from build123d import *

# Parameters (mm, degrees)
SALIENTE_EXTRUIR3_DEPTH    = 3
SALIENTE_EXTRUIR4_DEPTH    = 37
CROQUIS15_R                = 1.05
CROQUIS15_W                = 14
CROQUIS15_H                = 5.5
CORTAR_EXTRUIR6_DEPTH      = 9
CROQUIS17_W                = 2.75
CROQUIS17_H                = 14
CROQUIS17_R                = 1.05
CORTAR_EXTRUIR7_DEPTH      = 205.947432284
CORTAR_EXTRUIR8_DEPTH      = 200.161793525
CORTAR_EXTRUIR8_DEPTH_BACK = 200.161793525
CROQUIS18_R                = 4.05
CROQUIS18_R_2              = 1.55
CROQUIS20_R                = 1.55
CROQUIS20_R_2              = 4.05
CORTAR_EXTRUIR9_DEPTH      = 5.5
CROQUIS21_W                = 38.703075187
CROQUIS21_H                = 31.902541418
CROQUIS21_R                = 1.55
CROQUIS21_R_2              = 4.05
CORTAR_EXTRUIR11_DEPTH     = 5.5
CROQUIS24_R                = 1.55
CORTAR_EXTRUIR12_DEPTH     = 5.5
SALIENTE_EXTRUIR5_START    = 5.5
CROQUIS25_R                = 3.5
CROQUIS25_R_2              = 1.55
SALIENTE_EXTRUIR5_DEPTH    = 5.5
CROQUIS27_W                = 4.4
CROQUIS27_H                = 9.7
CORTAR_EXTRUIR13_DEPTH     = 191.373895269
CROQUIS28_R                = 1.55
CORTAR_EXTRUIR14_DEPTH     = 5.5


with BuildPart() as part:
    # PacmanSilueta → Saliente-Extruir3 (new body)
    with BuildSketch(Plane.XY):
        Polygon((-79.1, 2.1), (-79.1, -93), (-79.1, -100.1), (-68.1, -100.1), (-68.1, -111.1), (-31.486400432, -111.1), (-31.486400432, -100.1), (-13.1, -100.1), (-13.1, -111.1), (23.1, -111.1), (23.1, -100.1), (41.486400432, -100.1), (41.486400432, -111.1), (78.1, -111.1), (78.1, -100.1), (89.1, -100.1), (89.1, 2.1), (78.1, 2.1), (78.1, 35.1), (67.1, 35.1), (67.1, 46.1), (56.1, 46.1), (56.1, 57.1), (34.1, 57.1), (34.1, 68.1), (-24.1, 68.1), (-24.1, 57.1), (-46.1, 57.1), (-46.1, 46.1), (-57.1, 46.1), (-57.1, 35.1), (-68.1, 35.1), (-68.1, 2.1), align=None)
    extrude(amount=-SALIENTE_EXTRUIR3_DEPTH)

    # Croquis3 → Saliente-Extruir4 (add)
    with BuildSketch(Plane.XY):
        Polygon((-46.1, 46.1), (-57.1, 46.1), (-57.1, 35.1), (-68.1, 35.1), (-68.1, 2.1), (-79.1, 2.1), (-79.1, -100.1), (-68.1, -100.1), (-68.1, -111.1), (-31.486400432, -111.1), (-31.486400432, -100.1), (-13.1, -100.1), (-13.1, -111.1), (23.1, -111.1), (23.1, -100.1), (41.486400432, -100.1), (41.486400432, -111.1), (78.1, -111.1), (78.1, -100.1), (89.1, -100.1), (89.1, 2.1), (78.1, 2.1), (78.1, 35.1), (67.1, 35.1), (67.1, 46.1), (56.1, 46.1), (56.1, 57.1), (34.1, 57.1), (34.1, 68.1), (-24.1, 68.1), (-24.1, 57.1), (-46.1, 57.1), align=None)
        Polygon((-72, -93), (-72, -5), (-61, -5), (-61, 28), (-50, 28), (-50, 39), (-39, 39), (-39, 50), (-17, 50), (-17, 61), (27, 61), (27, 50), (49, 50), (49, 39), (60, 39), (60, 28), (71, 28), (71, -5), (82, -5), (82, -93), (71, -93), (71, -104), (48.586400432, -104), (48.586400432, -93), (16, -93), (16, -104), (-6, -104), (-6, -93), (-38.586400432, -93), (-38.586400432, -104), (-61, -104), (-61, -93), align=None, mode=Mode.SUBTRACT)
    extrude(amount=SALIENTE_EXTRUIR4_DEPTH)

    # Croquis15 → Cortar-Extruir6 (cut)
    with BuildSketch(Plane(origin=(0, 68.1, 0), x_dir=(1, 0, 0), z_dir=(0, 1, 0))):
        with Locations(Location((-15.4, -8.6, 0), (0, 0, 180))):
            Circle(CROQUIS15_R)
        with Locations((-15.4, -25.4)):
            Circle(CROQUIS15_R)
        with Locations(Location((25.4, -8.6, 0), (0, 0, 180))):
            Circle(CROQUIS15_R)
        with Locations(Location((25.4, -25.4, 0), (0, 0, 180))):
            Circle(CROQUIS15_R)
        with Locations((5, -7)):
            Rectangle(CROQUIS15_W, CROQUIS15_H)
    extrude(amount=-CORTAR_EXTRUIR6_DEPTH, mode=Mode.SUBTRACT)

    # Croquis17 → Cortar-Extruir7 (cut, through all)
    with BuildSketch(Plane.ZY.offset(79.1)):
        with Locations((8.375, -29)):
            Rectangle(CROQUIS17_W, CROQUIS17_H)
        with Locations((5.625, -29)):
            Rectangle(CROQUIS17_W, CROQUIS17_H)
        with Locations((25.4, -8.6)):
            Circle(CROQUIS17_R)
        with Locations(Location((8.6, -8.6, 0), (0, 0, 180))):
            Circle(CROQUIS17_R)
        with Locations(Location((25.4, -49.4, 0), (0, 0, 180))):
            Circle(CROQUIS17_R)
        with Locations((8.6, -49.4)):
            Circle(CROQUIS17_R)
    extrude(amount=-CORTAR_EXTRUIR7_DEPTH, mode=Mode.SUBTRACT)

    # Croquis18 → Cortar-Extruir8 (cut, two sides: drawn at the far end of the back side and taken through both)
    with BuildSketch(Plane(origin=(-72, 0, 0), x_dir=(0, 0, -1), z_dir=(1, 0, 0)).offset(-CORTAR_EXTRUIR8_DEPTH_BACK)):
        with Locations((-19.5, -75.903746181)):
            Circle(CROQUIS18_R)
        with Locations((-19.5, -67.303746181)):
            Circle(CROQUIS18_R_2)
        with Locations((-19.5, -84.503746181)):
            Circle(CROQUIS18_R_2)
    extrude(amount=CORTAR_EXTRUIR8_DEPTH + CORTAR_EXTRUIR8_DEPTH_BACK, mode=Mode.SUBTRACT)

    # Croquis20 → Cortar-Extruir9 (cut)
    with BuildSketch(Plane(origin=(-72, 0, 0), x_dir=(0, 0, -1), z_dir=(1, 0, 0))):
        Polygon((0, -90.222340764), (0, -75.903746181), (0, -64.555188751), (0, -61.906996068), (-39.638162785, -61.906996068), (-39.638162785, -90.222340764), align=None)
        with Locations((-19.5, -84.503746181)):
            Circle(CROQUIS20_R, mode=Mode.SUBTRACT)
        with Locations((-19.5, -75.903746181)):
            Circle(CROQUIS20_R_2, mode=Mode.SUBTRACT)
        with Locations((-19.5, -67.303746181)):
            Circle(CROQUIS20_R, mode=Mode.SUBTRACT)
    extrude(amount=-CORTAR_EXTRUIR9_DEPTH, mode=Mode.SUBTRACT)

    # Croquis21 → Cortar-Extruir11 (cut)
    with BuildSketch(Plane.ZY.offset(-82)):
        with Locations((19.351537594, -75.274989688)):
            Rectangle(CROQUIS21_W, CROQUIS21_H)
        with Locations(Location((19.5, -84.503746181, 0), (0, 0, 270))):
            Circle(CROQUIS21_R, mode=Mode.SUBTRACT)
        with Locations(Location((19.5, -75.903746181, 0), (0, 0, 180))):
            Circle(CROQUIS21_R_2, mode=Mode.SUBTRACT)
        with Locations(Location((19.5, -67.303746181, 0), (0, 0, 180))):
            Circle(CROQUIS21_R, mode=Mode.SUBTRACT)
    extrude(amount=-CORTAR_EXTRUIR11_DEPTH, mode=Mode.SUBTRACT)

    # Croquis24 → Cortar-Extruir12 (cut)
    with BuildSketch(Plane.XY):
        with Locations((26.294334913, 22.504861365)):
            Circle(CROQUIS24_R)
        with Locations((-55.705665087, -14.495138635)):
            Circle(CROQUIS24_R)
        with Locations((65.6, -67.464668416)):
            Circle(CROQUIS24_R)
        with Locations((26.294334913, -14.495138635)):
            Circle(CROQUIS24_R)
        with Locations((-55.705665087, 22.504861365)):
            Circle(CROQUIS24_R)
        with Locations((-69.8, -67.464668416)):
            Circle(CROQUIS24_R)
        with Locations((-55.6, -67.464668416)):
            Circle(CROQUIS24_R)
        with Locations((-55.6, -84.664668416)):
            Circle(CROQUIS24_R)
        with Locations((-69.8, -84.664668416)):
            Circle(CROQUIS24_R)
        with Locations((79.8, -67.464668416)):
            Circle(CROQUIS24_R)
        with Locations((79.8, -84.664668416)):
            Circle(CROQUIS24_R)
        with Locations((65.6, -84.664668416)):
            Circle(CROQUIS24_R)
    extrude(amount=-CORTAR_EXTRUIR12_DEPTH, mode=Mode.SUBTRACT)

    # Croquis25 → Saliente-Extruir5 (add)
    # profile 1 of 4: a face of its own
    with BuildSketch(Plane.XY.offset(SALIENTE_EXTRUIR5_START)):
        with Locations((-55.705665087, -14.495138635)):
            Circle(CROQUIS25_R)
        with Locations((-55.705665087, -14.495138635)):
            Circle(CROQUIS25_R_2, mode=Mode.SUBTRACT)
    # profile 2 of 4: a face of its own
    with BuildSketch(Plane.XY.offset(SALIENTE_EXTRUIR5_START)):
        with Locations((-55.705665087, 22.504861365)):
            Circle(CROQUIS25_R)
        with Locations((-55.705665087, 22.504861365)):
            Circle(CROQUIS25_R_2, mode=Mode.SUBTRACT)
    # profile 3 of 4: a face of its own
    with BuildSketch(Plane.XY.offset(SALIENTE_EXTRUIR5_START)):
        with Locations((26.294334913, 22.504861365)):
            Circle(CROQUIS25_R)
        with Locations((26.294334913, 22.504861365)):
            Circle(CROQUIS25_R_2, mode=Mode.SUBTRACT)
    # profile 4 of 4: a face of its own
    with BuildSketch(Plane.XY.offset(SALIENTE_EXTRUIR5_START)):
        with Locations((26.294334913, -14.495138635)):
            Circle(CROQUIS25_R)
        with Locations((26.294334913, -14.495138635)):
            Circle(CROQUIS25_R_2, mode=Mode.SUBTRACT)
    extrude(amount=-SALIENTE_EXTRUIR5_DEPTH)

    # Croquis27 → Cortar-Extruir13 (cut, through all)
    with BuildSketch(Plane(origin=(-61, 0, 0), x_dir=(0, 0, -1), z_dir=(1, 0, 0))):
        with Locations((-28.5, 4)):
            Rectangle(CROQUIS27_W, CROQUIS27_H)
    extrude(amount=-CORTAR_EXTRUIR13_DEPTH, mode=Mode.SUBTRACT)

    # Croquis28 → Cortar-Extruir14 (cut)
    with BuildSketch(Plane.XY.offset(37)):
        with Locations((5, -107.55)):
            Circle(CROQUIS28_R)
        with Locations((5, 64.55)):
            Circle(CROQUIS28_R)
        with Locations((85.55, -22.670703526)):
            Circle(CROQUIS28_R)
        with Locations((-75.55, -22.670703526)):
            Circle(CROQUIS28_R)
        with Locations((-57.1, 31.55)):
            Circle(CROQUIS28_R)
        with Locations((67.1, 31.55)):
            Circle(CROQUIS28_R)
        with Locations((-64.55, -107.55)):
            Circle(CROQUIS28_R)
        with Locations((74.55, -107.55)):
            Circle(CROQUIS28_R)
    extrude(amount=-CORTAR_EXTRUIR14_DEPTH, mode=Mode.SUBTRACT)


solid = part.part
Source: CAD feature listing. Evaluate the final solid. Frame: model axes, mm. A direction names the side the tool comes from. Give positions to 0.01 mm unless a question says otherwise; leave off trailing zeros. Write each loop counter-clockwise with the first axis right and the second up, starting at its lowest first coordinate (ties: lowest second). Pieces come first, ordered by that corner, then holes. Notation, with made-up numbers: M 61,-16 L 119,-16 A16 ccw 119,15 Z; hole C 65.25,1.5 d5. An arc over 180 degrees is marked long. Return JSON: item names as keys, results as strings. Group by question number.
1) Pull-direction query (Y, two-part tool) for faces 5 (the face through (-74, -100.1, 17)), 6 (the face through (84, 2.1, 17)), 7 (the face through (5, 65, 4.25)), 8 (the face through (29.63, 23.56, 2.79)); classes: pulls with the +Y half, pulls with the -Y half, needs draft (parallel to the pull), parting line crosses it, or undercut.
2) Cut plane A-A, the plane y = -32. Output: boundary loops of the cut face in (x, z), plus the area to 3 significant figures.
3) Cut plane C-C, the plane x = -27. Output: boundary loops of the cut face in (y, z), plus the area to 3 significant figures.
4) Set-up query: faces 1 (the face through (28, 22, 5.5)), 2 (the face through (23.1, -106, 17)), 3 (the face through (56.1, 52, 17)), 4 (the face through (-63, 35.1, 17)). Return all of +Z, -Z, +X, -X, +Y, -Y with unobstructed straight access to the full face (end or side cutting, diameter ignored); none if empty.
5) Material intervals for line 1 along X through (y, z) = (-101, 18.5); line 2 along Y through (x, z) = (-69.8, -1.1); line 3 along X through (y, z) = (-77.5, 31.5), sorted ascending. Write a range as [from, to].
6) Pin query (flat end, axial travel): P1, Ø9, axis at y = 44.5, z = 17.5, coming from the -X side; P2, Ø5, axis at y = -84.5, z = 19.5, coming from the -X side; P3, Ø9, axis at x = 32.5, z = 12.5, coming from the -Y side; P4, Ø1.5, axis at x = -28.5, z = 10.5, coming from the +Y side. Return the tip coordinate at first contact, or that it passes through.
7) Cut plane B-B, the plane x = 20.5. Output: boundary loops of the cut face in (y, z), plus the area to 3 significant figures.
Recorded:
{
 "1": {"face 5": "pulls with the -Y half", "face 6": "pulls with the +Y half", "face 7": "needs draft", "face 8": "undercut"},
 "2": {"outline": "M -79.1,-3 L 89.1,-3 L 89.1,4.25 L 82,4.25 L 82,0 L -72,0 L -72,4.25 L -79.1,4.25 Z; M -79.1,9.75 L -72,9.75 L -72,37 L -79.1,37 Z; M 82,9.75 L 89.1,9.75 L 89.1,37 L 82,37 Z", "area": "952 mm²"},
 "3": {"outline": "M -100.1,-3 L 57.1,-3 L 57.1,37 L 50,37 L 50,0 L -93,0 L -93,37 L -100.1,37 Z", "area": "997 mm²"},
 "4": {"face 1": "+Z", "face 2": "+Z, -Z, -Y", "face 3": "+Z, -Z, +X, +Y", "face 4": "+Z, -Z, -X, +Y"},
 "5": {"line 1": "x = [-68.1, -61], [-38.59, -31.49], [-13.1, -6], [16, 23.1], [41.49, 48.59], [71, 78.1]", "line 2": "y = [-100.1, -86.21], [-83.11, -69.01], [-65.91, 2.1]", "line 3": "x = [-79.1, -77.5], [87.5, 89.1]"},
 "6": {"P1": "stops at x = -57.1", "P2": "stops at x = -79.1", "P3": "stops at y = -100.1", "P4": "stops at y = 57.1"},
 "7": {"outline": "M -111.1,-3 L 68.1,-3 L 68.1,37 L 61,37 L 61,0 L -93,0 L -93,37 L -111.1,37 Z", "area": "1,470 mm²"}
}
